```python
from build123d import *

# Parameters (mm, degrees)
SKETCH_W         = 3.9
SKETCH_H         = 3.9
PAD_DEPTH        = 40
CHAMFER_SIZE2    = 3
CHAMFER_SIZE     = 30
CHAMFER001_SIZE  = 0.5
SKETCH001_W      = 3.9
SKETCH001_H      = 15
PAD001_DEPTH     = 3
CHAMFER002_SIZE2 = 2.9
CHAMFER002_SIZE  = 1
CHAMFER003_SIZE2 = 2.9
CHAMFER003_SIZE  = 1
CHAMFER004_SIZE2 = 2.9
CHAMFER004_SIZE  = 5
CHAMFER005_SIZE2 = 2.9
CHAMFER005_SIZE  = 5


with BuildPart() as part:
    # Sketch → Pad (new body)
    with BuildSketch(Plane.XY):
        with Locations((1.95, 1.95)):
            Rectangle(SKETCH_W, SKETCH_H)
    extrude(amount=PAD_DEPTH)

    # Chamfer
    chamfer_edges = [part.edges().sort_by_distance(p)[0] for p in [
        (3.9, 1.95, 40),
    ]]
    chamfer_side = part.faces().sort_by_distance((3.9, 1.95, 20))[0]
    chamfer(chamfer_edges, length=CHAMFER_SIZE, length2=CHAMFER_SIZE2, reference=chamfer_side)

    # Chamfer001
    chamfer001_edges = [part.edges().sort_by_distance(p)[0] for p in [
        (1.95, 0, 0),
        (3.9, 1.95, 0),
        (1.95, 3.9, 0),
        (0, 1.95, 0),
    ]]
    chamfer(chamfer001_edges, length=CHAMFER001_SIZE)

    # Sketch001 (on Face5 of Chamfer001) → Pad001 (join)
    with BuildSketch(Plane(origin=(0, 0, 0), x_dir=(0, -1, 0), z_dir=(-1, 0, 0))):
        with Locations((-1.95, 32.5)):
            Rectangle(SKETCH001_W, SKETCH001_H)
    extrude(amount=PAD001_DEPTH)

    # Chamfer002
    chamfer002_edges = [part.edges().sort_by_distance(p)[0] for p in [
        (-3, 3.9, 32.5),
    ]]
    chamfer002_side = part.faces().sort_by_distance((-3, 1.95, 32.5))[0]
    chamfer(chamfer002_edges, length=CHAMFER002_SIZE, length2=CHAMFER002_SIZE2, reference=chamfer002_side)

    # Chamfer003
    chamfer003_edges = [part.edges().sort_by_distance(p)[0] for p in [
        (-3, 0, 32.5),
    ]]
    chamfer003_side = part.faces().sort_by_distance((-3, 1.45, 32.5))[0]
    chamfer(chamfer003_edges, length=CHAMFER003_SIZE, length2=CHAMFER003_SIZE2, reference=chamfer003_side)

    # Chamfer004
    chamfer004_edges = [part.edges().sort_by_distance(p)[0] for p in [
        (-3, 1.95, 40),
    ]]
    chamfer004_side = part.faces().sort_by_distance((-3, 1.95, 32.5))[0]
    chamfer(chamfer004_edges, length=CHAMFER004_SIZE, length2=CHAMFER004_SIZE2, reference=chamfer004_side)

    # Chamfer005
    chamfer005_edges = [part.edges().sort_by_distance(p)[0] for p in [
        (-3, 1.95, 25),
    ]]
    chamfer005_side = part.faces().sort_by_distance((-3, 1.95, 30))[0]
    chamfer(chamfer005_edges, length=CHAMFER005_SIZE, length2=CHAMFER005_SIZE2, reference=chamfer005_side)


solid = part.part
```
Build history of the part. All positions in model axes, mm. A direction names the side the tool comes from. Round coordinates to 2 decimals unless told otherwise and drop trailing zeros. Write each loop counter-clockwise with the first axis right and the second up, starting at its lowest first coordinate (ties: lowest second). Pieces come first, ordered by that corner, then holes.
1) Band-saw the part on A-A, the plane x = 2.5. List the corners of the cut face in (y, z).
2) 3-axis set-ups, long thin cutter, end or side, ignore diameter. For faces 1 (the flat face through (0, 2, 13)), 2 (the flat face through (2.38, 1.92, 25.21)): which of +Z, -Z, +X, -X, +Y, -Y reach the whole face in a straight line?
3) Pin check, flat tip, straight feed: pin 1 (1 mm diameter, centred on y = 0.5, z = 11.5, fed in from -X). Stop position of the tip, or through.
4) Drill centre lines: probe 1 along X at (y, z) = (3.5, 2.5); probe 2 along Z at (x, y) = (0.25, 1.5); probe 3 along X at (y, z) = (2, 16). Where is each one in solid material? Low to high.
5) Band-saw the part on D-D, the plane z = 17.5. List the corners of the cut face in (x, y).
6) Band-saw the part on B-B, the plane z = 26.5. List the corners of the cut face in (x, y), and give its area (3 significant figures).
7) Band-saw the part on C-C, the plane y = 1.35. List the corners of the cut face in (x, z), and give its area (3 significant figures).
Ans:
1. outline: (0, 0.5) - (0.5, 0) - (3.4, 0) - (3.9, 0.5) - (3.9, 24) - (0, 24) - close
2. face 1: -Z, -X, +Y, -Y
2. face 2: +Z, +X, +Y, -Y
3. pin 1: stops at x = 0
4. probe 1: x = 0 to 3.9
4. probe 2: z = 0.25 to 40
4. probe 3: x = 0 to 3.3
5. outline: (0, 0) - (3.15, 0) - (3.15, 3.9) - (0, 3.9) - close
6. outline: (-0.97, 0.3) - (-0.1, 0) - (2.25, 0) - (2.25, 3.9) - (-0.1, 3.9) - (-0.97, 3.6) - close
6. area: 12.3 mm2
7. outline: (-3, 30) - (-0.1, 25) - (0, 25) - (0, 0.5) - (0.5, 0) - (3.4, 0) - (3.9, 0.5) - (3.9, 10) - (0.9, 40) - (-0.1, 40) - (-3, 35) - close
7. area: 141 mm2
